Model file for the job. Use its own axes, mm. Round coordinates to 2 decimals unless told otherwise and drop trailing zeros. Loops run counter-clockwise (first coordinate to the right, second up) from the corner with the lowest first, then second, coordinate; pieces in that order, holes last. Notation, with made-up numbers: (59.5, -27.5) - (78.5, -27.5) arc R28 ccw to (78.5, -8.5) - close; hole circle Ø6 at (-31.5, 0.25). An arc over 180 degrees is marked (long way). Use one line per item in the form item = value.
Autodesk Inventor part; units mm, degrees
ref_plane "Work Plane1" through (0, 11, 0) normal (0, 1, 0) x (-1, 0, 0)
ref_plane "YZ Plane" through (0, 0, 0) normal (1, 0, 0) x (0, 1, 0)
ref_plane "XY Plane" through (0, 0, 0) normal (0, 0, 1) x (1, 0, 0)
sketch "Sketch1" plane through (0, 0, 0) normal (1, 0, 0) x (0, 1, 0)
  circle A0 centre (0, 0) radius 11
  circle A1 centre (0, 0) radius 5
  dimension "d0" = 22
  dimension "d1" = 10
extrude "Extrusion1" add sketch "Sketch1" along normal blind 50
ref_plane "Work Plane1" through (0, 11, 0) normal (0, 1, 0) x (-1, 0, 0)
sketch "Sketch2" plane through (0, 11, 0) normal (0, 1, 0) x (-1, 0, 0)
  circle A0 centre (-9, 0) radius 7.6
  point P0 (0, 0)
  dimension "d5" = 15.2
  dimension "d6" = 9
extrude "Extrusion2" add sketch "Sketch2" along normal blind 7.2 and the other way blind 5
properties part number "sample-transfer_shuttle-mockup"
1. Flat gauge pins, fed straight in: pin 1 (2 mm diameter, centred on x = 8, y = -2.5, fed in from +Z); pin 2 (4 mm diameter, centred on x = 38, y = -5, fed in from +Z); pin 3 (8 mm diameter, centred on x = 43.5, z = -4.5, fed in from +Y). Where does each tip first touch, or does it go through?
Geometry check:
pin_1 = 10.9
pin_2 = 10.58
pin_3 = 10.99
2. Cut at A-A, the plane z = 0. Give the cut face in (x, y).
Geometry check:
outline = (0, -11) - (50, -11) - (50, -5) - (0, -5) - close; (0, 5) - (50, 5) - (50, 11) - (16.6, 11) - (16.6, 18.2) - (1.4, 18.2) - (1.4, 11) - (0, 11) - close
3. Cut at D-D, the plane y = 10. Give the cut face in (x, z), plus the area to 3 significant figures.
Geometry check:
outline = (0, -4.58) - (2.94, -4.58) arc R7.6 ccw to (15.06, -4.58) - (50, -4.58) - (50, 4.58) - (15.06, 4.58) arc R7.6 ccw to (2.94, 4.58) - (0, 4.58) - close
area = 509 mm^2
4. Cut at C-C, the plane y = 0. Give the cut face in (x, z).
Geometry check:
outline = (0, -11) - (50, -11) - (50, -5) - (0, -5) - close; (0, 5) - (50, 5) - (50, 11) - (0, 11) - close
5. Wall check: probe 1 along Z at (x, y) = (30, 0); probe 2 along Y at (x, z) = (4.5, 3); probe 3 along Y at (x, z) = (12.5, -2). Give the ranges that are in metal, low to high.
Geometry check:
probe_1 = -11 to -5, 5 to 11
probe_2 = -10.58 to -4, 4 to 18.2
probe_3 = -10.82 to -4.58, 4.58 to 18.2
6. Cut at B-B, the plane x = 9. Give the cut face in (y, z), plus the area to 3 significant figures.
Geometry check:
outline = (7.95, -7.6) - (18.2, -7.6) - (18.2, 7.6) - (7.95, 7.6) arc R11 ccw (long way) to start; hole circle Ø10 at (0, 0)
area = 426 mm^2
7. Pull direction Z, two halves, no side cores. Call faces 1 (the cylindrical face through (4.9, 14.3, 6.4)), 2 (the flat face through (9, 18.2, 0)), 3 (the cylindrical face through (24.65, -1.08, 4.88)): +Z half, -Z half, draft (parallel to the pull), parting line (faces both ways), or undercut.
Geometry check:
face_1 = parting line
face_2 = draft
face_3 = undercut
